Input: part model. Units: mm. Frame: model coordinates. Round coordinates to 2 decimals unless told otherwise and drop trailing zeros. Loops run counter-clockwise (first coordinate to the right, second up) from the corner with the lowest first, then second, coordinate; pieces in that order, holes last. Notation, with made-up numbers: M -29,-16 L 29,-16 A25 ccw 29,-2 Z; hole C 3,-21 d11. An arc over 180 degrees is marked long. Return JSON: item names as keys, results as strings. Group by question number.
1) Section B-B (z = 0). Output: boundary loops of the cut face in (x, y).
2) Material intervals for line 1 (Y direction, x = 51.85, z = 0); line 2 (X direction, y = 0.1, z = 0); line 3 (X direction, y = 2.75, z = -12), sorted ascending. Write a range as from..to.
3) Contact query for flat-ended pins moving along their axis: P1, Ø1, axis at x = -16.5, y = 3.5, coming from the +Z side; P2, Ø3, axis at y = 3, z = 0, coming from the +X side; P3, Ø1.5, axis at y = 3.5, z = 26, coming from the -X side. Output: stop coordinate, or through.
4) Section A-A (x = 0). Output: boundary loops of the cut face in (y, z).
from build123d import *

# Parameters (mm, degrees)
SKETCH1_R                 = 53.25
SKETCH1_R_2               = 48.5
BOSS_EXTRUDE1_DEPTH       = 6
SKETCH3_R                 = 2.85
SKETCH4_R                 = 2.5
CUT_EXTRUDE1_DEPTH        = 120
CUT_EXTRUDE2_REACH        = 78.046
CUT_EXTRUDE2_START_RADIUS = 53.25
CUT_EXTRUDE2_END_RADIUS   = 53.25
SKETCH6_W                 = 1.240344628
SKETCH6_H                 = 0.651674146


with BuildPart() as part:
    # Sketch1 → Boss-Extrude1 (new body)
    with BuildSketch(Plane(origin=(0, 0, 0), x_dir=(1, 0, 0), z_dir=(0, 1, 0))):
        with Locations(Location((0, 0, 0), (0, 0, 270))):
            Circle(SKETCH1_R)
        with Locations(Location((0, 0, 0), (0, 0, 270))):
            Circle(SKETCH1_R_2, mode=Mode.SUBTRACT)
    extrude(amount=BOSS_EXTRUDE1_DEPTH)

    # Sketch3 → Cut-Revolve1 (revolve, cut)
    with BuildSketch(Plane.XY, mode=Mode.PRIVATE) as cut_revolve1_sk:
        with Locations((-47.7, 3)):
            Circle(SKETCH3_R)
    revolve(cut_revolve1_sk.sketch.rotate(Axis((0, 0, 0), (0, 1, 0)), 270), axis=Axis((0, 0, 0), (0, 1, 0)), mode=Mode.SUBTRACT)

    # Sketch4 → Cut-Extrude1 (cut)
    with BuildSketch(Plane(origin=(0, 0, 0), x_dir=(0, 0, -1), z_dir=(1, 0, 0))):
        with Locations(Location((0, 3, 0), (0, 0, 180))):
            Circle(SKETCH4_R)
    extrude(amount=CUT_EXTRUDE1_DEPTH, mode=Mode.SUBTRACT)

    # Cut-Extrude2: from a cylinder face, 78.046 long prism both ways, kept between that surface and its translate by the depth
    cut_extrude2_start = Plane(origin=(0, 3, 0), z_dir=(0, -1, 0)) * Cylinder(CUT_EXTRUDE2_START_RADIUS, 263.592, mode=Mode.PRIVATE)
    cut_extrude2_end = Plane(origin=(-0.5, 3, 0), z_dir=(0, -1, 0)) * Cylinder(CUT_EXTRUDE2_END_RADIUS, 263.592, mode=Mode.PRIVATE)
    # Sketch6 → Cut-Extrude2 (cut, from a surface)
    with BuildSketch(Plane(origin=(0, 0, 0), x_dir=(0, 0, -1), z_dir=(1, 0, 0)), mode=Mode.PRIVATE) as cut_extrude2_sk1:
        with Locations((3.176747556, 3)):
            Rectangle(SKETCH6_W, SKETCH6_H)
    cut_extrude2_tool1 = extrude(cut_extrude2_sk1.sketch, amount=CUT_EXTRUDE2_REACH, both=True, mode=Mode.PRIVATE)
    add(((cut_extrude2_tool1 & cut_extrude2_start) - cut_extrude2_end).solids().sort_by_distance((52.901527, 3, -3.176748))[0], mode=Mode.SUBTRACT)


solid = part.part
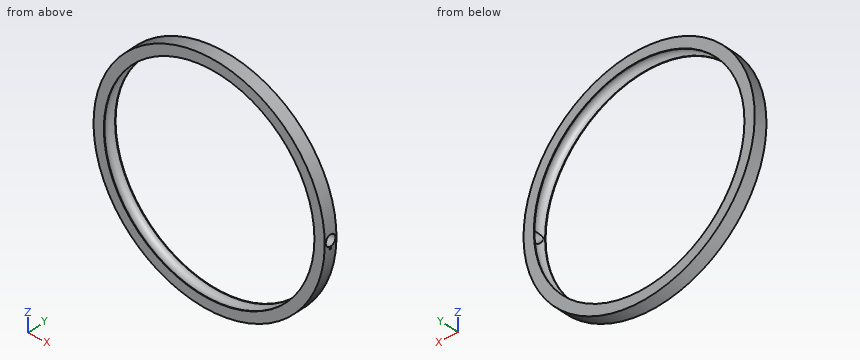
Returned:
{
 "1": {"outline": "M -53.25,0 L -48.5,0 L -48.5,0.26 A2.85 cw -48.5,5.74 L -48.5,6 L -53.25,6 Z; M 48.5,0 L 53.25,0 L 53.25,0.5 L 49.07,0.5 A2.85 cw 48.5,0.26 Z; M 48.5,5.74 A2.85 cw 49.07,5.5 L 53.25,5.5 L 53.25,6 L 48.5,6 Z"},
 "2": {"line 1": "y = 0..0.5, 5.5..6", "line 2": "x = -53.25..-48.5, 48.5..53.25", "line 3": "x = -51.88..-49.09, 49.09..51.88"},
 "3": {"P1": "stops at z = 50.79", "P2": "stops at x = -50.12", "P3": "stops at x = -46.88"},
 "4": {"outline": "M 0,-53.25 L 6,-53.25 L 6,-48.5 L 5.74,-48.5 A2.85 cw 0.26,-48.5 L 0,-48.5 Z; M 0,48.5 L 0.26,48.5 A2.85 cw 5.74,48.5 L 6,48.5 L 6,53.25 L 0,53.25 Z"}
}
